Verification items for this drawing (mm, ordinates from the low corner). Coordinates: 2 decimals unless noted, no trailing zeros. Order: outer loops, then holes, each group sorted by start corner. A loop starts at its lowest first (then second) coordinate and runs counter-clockwise, first axis right, second up. Notation, with made-up numbers: M 78.5,12 L 87.5,12 A22 cw 87.5,34 Z; hole C -30.75,51 d3. An arc over 180 degrees is marked long. One line per item, written item: value. Start each with the question number.
1) Sectioned sample at D-D, the plane z = 42. Enter the section's corners in (x, y), then the cut area to 3 significant figures.
2) Sectioned sample at C-C, the plane x = 82. Enter the section's corners in (y, z), then the cut area to 3 significant figures.
3) Sectioned sample at B-B, the plane y = 2.1. Enter the section's corners in (x, z), then the cut area to 3 significant figures.
4) Go/stop test with flat-tipped pins: P1, Ø3, axis at x = 82, z = 42, coming from the +Y side; P2, Ø1.5, axis at x = 57.5, y = 1, coming from the +Z side. Record where each tip stops, or that it passes through.
5) Sectioned sample at A-A, the plane z = 10. Enter the section's corners in (x, y).
6) Thickness scan on L1, parallel to Z at x = 10, y = 2.1; L2, parallel to X at y = 1.2, z = 10; L3, parallel to X at y = 2.15, z = 42. Record the ranges inside material, lowest first. Write a range as from..to.
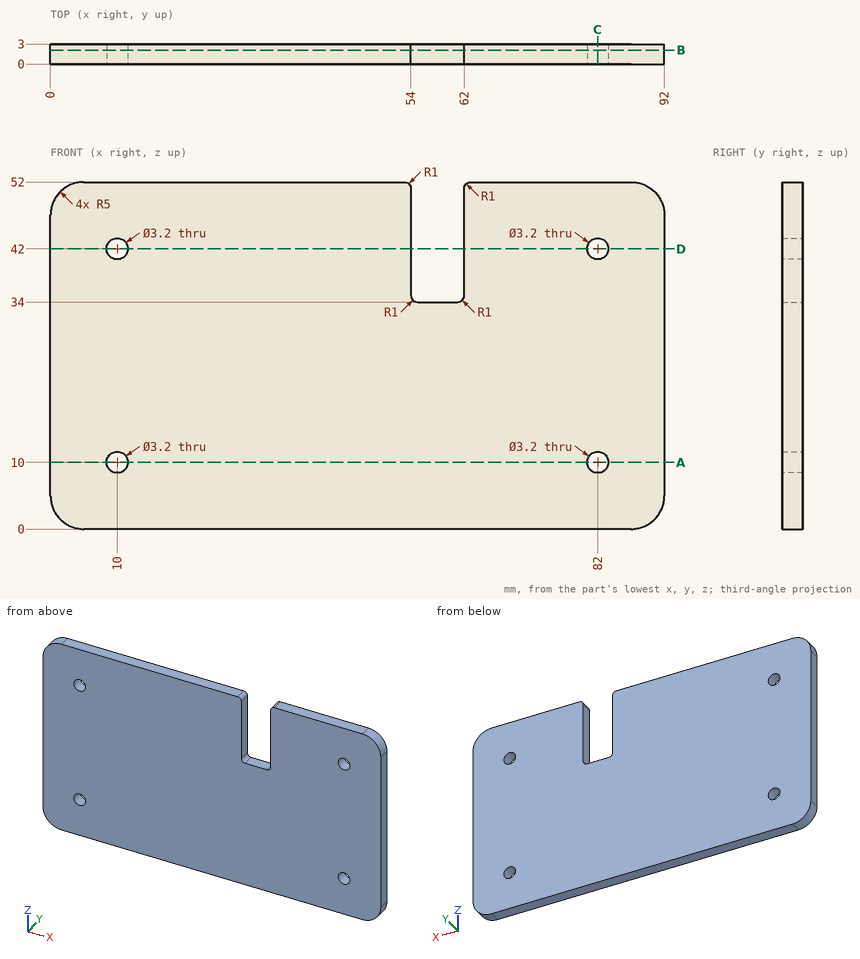
Final values:
1. outline: M 0,0 L 8.4,0 L 8.4,3 L 0,3 Z; M 11.6,0 L 54,0 L 54,3 L 11.6,3 Z; M 62,0 L 80.4,0 L 80.4,3 L 62,3 Z; M 83.6,0 L 92,0 L 92,3 L 83.6,3 Z
1. area: 233 mm^2
2. outline: M 0,0 L 3,0 L 3,8.4 L 0,8.4 Z; M 0,11.6 L 3,11.6 L 3,40.4 L 0,40.4 Z; M 0,43.6 L 3,43.6 L 3,52 L 0,52 Z
2. area: 137 mm^2
3. outline: M 0,5 A5 ccw 5,0 L 87,0 A5 ccw 92,5 L 92,47 A5 ccw 87,52 L 63,52 A1 ccw 62,51 L 62,35 A1 cw 61,34 L 55,34 A1 cw 54,35 L 54,51 A1 ccw 53,52 L 5,52 A5 ccw 0,47 Z; hole C 10,10 d3.2; hole C 10,42 d3.2; hole C 82,10 d3.2; hole C 82,42 d3.2
3. area: 4,590 mm^2
4. P1: passes through
4. P2: stops at z = 34
5. outline: M 0,0 L 8.4,0 L 8.4,3 L 0,3 Z; M 11.6,0 L 80.4,0 L 80.4,3 L 11.6,3 Z; M 83.6,0 L 92,0 L 92,3 L 83.6,3 Z
6. L1: z = 0..8.4, 11.6..40.4, 43.6..52
6. L2: x = 0..8.4, 11.6..80.4, 83.6..92
6. L3: x = 0..8.4, 11.6..54, 62..80.4, 83.6..92
